For this review, take the finished solid that the model builds, in its own axes (mm). Give positions to 0.01 mm unless a question says otherwise; leave off trailing zeros. Write each loop counter-clockwise with the first axis right and the second up, starting at its lowest first coordinate (ties: lowest second). Pieces come first, ordered by that corner, then holes. Notation, with made-up numbers: (19, 35.25) -> (74, 35.25) arc R23 ccw to (74, 51.25) -> close; hole circle Ø9 at (10, -8.5). An arc over 180 degrees is marked (long way). Write item = value, one per line.
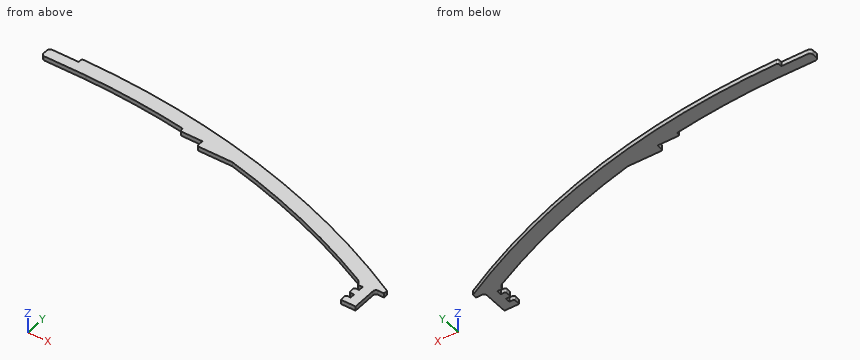
```python
from build123d import *

# Parameters (mm, degrees)
BOSS_EXTRUDE1_DEPTH = 1.5
SKETCH3_W           = 4.820379215
SKETCH3_H           = 3.3
CUT_EXTRUDE1_DEPTH  = 10
FILLET1_R           = 1
SKETCH4_W           = 2
SKETCH4_H           = 7.019019915
CUT_EXTRUDE2_DEPTH  = 10


with BuildPart() as part:
    # Sketch2 → Boss-Extrude1 (new, symmetric)
    with BuildSketch(Plane.XY):
        with BuildLine():
            Line((299.5, -67.353443934), (293.5, -67.353443934))
            ThreePointArc((293.5, -67.353443934), (292.085786438, -67.939230372), (291.5, -69.353443934))
            Line((291.5, -69.353443934), (291.5, -85.649534053))
            Line((291.5, -85.649534053), (281.5, -85.649534053))
            Line((281.5, -85.649534053), (281.5, -70.504592149))
            ThreePointArc((281.5, -70.504592149), (280.757064897, -67.882112699), (278.749040614, -66.038966065))
            ThreePointArc((278.749040614, -66.038966065), (222.498981863, -41.753539728), (163.781589842, -24.257285386))
            Line((163.781589842, -24.257285386), (141, -24.257285386))
            ThreePointArc((141, -24.257285386), (140.292893219, -23.964392167), (140, -23.257285386))
            Line((140, -23.257285386), (140, -19.257285386))
            Line((140, -19.257285386), (126, -19.257285386))
            ThreePointArc((126, -19.257285386), (125.292893219, -18.964392167), (125, -18.257285386))
            Line((125, -18.257285386), (125, -17.551725847))
            ThreePointArc((125, -17.551725847), (124.759050209, -16.900693759), (124.152314439, -16.563393762))
            ThreePointArc((124.152314439, -16.563393762), (89.724531973, -12.428170907), (55.097618142, -10.598112953))
            ThreePointArc((55.097618142, -10.598112953), (55.000467449, -10.596696958), (54.903307584, -10.596224945))
            Line((54.903307584, -10.596224945), (27, -10.596224945))
            ThreePointArc((27, -10.596224945), (25.585786438, -10.010438507), (25, -8.596224945))
            Line((25, -8.596224945), (25, -5.5))
            ThreePointArc((25, -5.5), (25.585786438, -4.085786438), (27, -3.5))
            Line((27, -3.5), (45, -3.5))
            Line((45, -3.5), (45, -1.500945781))
            ThreePointArc((45, -1.500945781), (45.293562303, -0.793170548), (46.001891561, -0.50094757))
            ThreePointArc((46.001891561, -0.50094757), (176.838494864, -17.170276226), (299.5, -65.649534053))
            Line((299.5, -65.649534053), (299.5, -67.353443934))
        make_face()
    extrude(amount=BOSS_EXTRUDE1_DEPTH, both=True)

    # Sketch3 → Cut-Extrude1 (cut)
    with BuildSketch(Plane.XY.offset(1.5)):
        with Locations((282.389810393, -71.353443934)):
            Rectangle(SKETCH3_W, SKETCH3_H)
        with Locations((282.389810393, -79.353443934)):
            Rectangle(SKETCH3_W, SKETCH3_H)
    extrude(amount=-CUT_EXTRUDE1_DEPTH, mode=Mode.SUBTRACT)

    # Fillet1
    fillet1_edges = [part.edges().sort_by_distance(p)[0] for p in [
        (281.435398823, -69.703443934, 0),
        (281.5, -73.003443934, 0),
        (281.5, -81.003443934, 0),
        (281.5, -77.703443934, 0),
    ]]
    fillet(fillet1_edges, radius=FILLET1_R)

    # Sketch4 → Cut-Extrude2 (cut)
    with BuildSketch(Plane.XY.offset(1.5)):
        with Locations((298.5, -66.105228371)):
            Rectangle(SKETCH4_W, SKETCH4_H)
    extrude(amount=-CUT_EXTRUDE2_DEPTH, mode=Mode.SUBTRACT)


solid = part.part
```
(1) For pin 1 (1.5 mm diameter, centred on x = 294.5, z = 0.5, fed in from -Y); pin 2 (0.9 mm diameter, centred on x = 44, z = 0.5, fed in from -Y); pin 3 (0.9 mm diameter, centred on x = 35.5, z = 0.5, fed in from +Y), all flat-tipped, find the tip position at first contact; note any pin that passes through.
Answers below:
pin_1 = -67.35
pin_2 = -10.6
pin_3 = -3.5
(2) To check wall thickness, follow probe 1 along Y at (x, z) = (58, 0.7); probe 2 along Y at (x, z) = (271.5, -0.4); probe 3 along X at (y, z) = (-69.5, 0.75). State the ranges of each line that lie inside material, in increasing order.
Answers below:
probe_1 = -10.66 to -0.66
probe_2 = -62.46 to -51.37
probe_3 = 281.62 to 291.5
(3) Take a section at A-A (x = 186.5). Write out the cut boundary in (y, z).
Answers below:
outline = (-30.14, -1.5) -> (-19.75, -1.5) -> (-19.75, 1.5) -> (-30.14, 1.5) -> close
(4) Take a section at B-B (y = -40.5). Write out the cut boundary in (x, z), plus the area to 3 significant figures.
Answers below:
outline = (219.01, -1.5) -> (246.92, -1.5) -> (246.92, 1.5) -> (219.01, 1.5) -> close
area = 83.7 mm^2
